Autodesk Inventor part; units mm, degrees
ref_plane "YZ Plane" through (0, 0, 0) normal (1, 0, 0) x (0, 1, 0)
ref_plane "XZ Plane" through (0, 0, 0) normal (0, 1, 0) x (-1, 0, 0)
ref_plane "XY Plane" through (0, 0, 0) normal (0, 0, 1) x (1, 0, 0)
sketch "Boceto1" plane through (0, 0, 0) normal (0, 1, 0) x (-1, 0, 0)
  line L0 (-50, 28) -> (-53, 28)
  line L1 (-50, -28) -> (-50, -22)
  line L2 (-50, -28) -> (-53, -28)
  circle A0 centre (-25, 0) radius 1.5
  circle A1 centre (25, 0) radius 1.5
  line L3 (-53, -25) -> (-53, -28)
  line L4 (-53, -22) -> (-53, -25)
  line L5 (-50, -22) -> (-53, -22)
  line L6 (-50, -28) -> (-50, -22)
  line L7 (-53, -25) -> (-53, -28)
  line L8 (-53, -22) -> (-53, -25)
  line L9 (53, 4.5) -> (53, -4.5)
  line L10 (50, 4.5) -> (53, 4.5)
  line L11 (50, -4.5) -> (50, 4.5)
  line L12 (53, -4.5) -> (50, -4.5)
  line L13 (-50, 22) -> (-50, 28)
  line L14 (-53, 22) -> (-50, 22)
  line L15 (-53, 28) -> (-53, 22)
  line L16 (-50, 28) -> (-53, 28)
  line L17 (19.5, 28) -> (19.5, 25)
  line L18 (6.5, 28) -> (19.5, 28)
  line L19 (6.5, 25) -> (6.5, 28)
  line L20 (19.5, 25) -> (6.5, 25)
  line L21 (56, 31) -> (56, -31)
  line L22 (-56, 31) -> (56, 31)
  line L23 (-56, -31) -> (-56, 31)
  line L24 (56, -31) -> (-56, -31)
  line L25 (-19.5, 28) -> (-19.5, 25)
  line L26 (-6.5, 28) -> (-19.5, 28)
  line L27 (-6.5, 25) -> (-6.5, 28)
  line L28 (-19.5, 25) -> (-6.5, 25)
  line L29 (-19.5, -28) -> (-19.5, -25)
  line L30 (-6.5, -28) -> (-19.5, -28)
  line L31 (-6.5, -25) -> (-6.5, -28)
  line L32 (-19.5, -25) -> (-6.5, -25)
  line L33 (19.5, -25) -> (19.5, -28)
  line L34 (6.5, -25) -> (19.5, -25)
  line L35 (6.5, -28) -> (6.5, -25)
  line L36 (19.5, -28) -> (6.5, -28)
extrude "Extrusión1" add sketch "Boceto1" along normal blind 3
properties part number "Case_Base2" material "MDF Tablero de fibras de densidad media"
Check sheet for the modelled part. Datum: model origin and axes. Units: mm. A direction names the side the tool comes from. Round coordinates to 2 decimals unless told otherwise and drop trailing zeros. Loops run counter-clockwise (first coordinate to the right, second up) from the corner with the lowest first, then second, coordinate; pieces in that order, holes last. Notation, with made-up numbers: M -24,24.25 L -19,24.25 A21 ccw -19,53.25 Z; hole C 4,14 d5. An arc over 180 degrees is marked long. Answer as a JSON object with one key per item and string values.
1. Section check B-B (y = 2.25). State how many separate pieces and enclosed holes the cut face has, plus the area to 3 significant figures.
Reply:
{"separate pieces": "1", "enclosed holes": "9", "area": "6,710 mm²"}
2. Scan lines: line 1 (Z direction, x = 11.5, y = 2.55); line 2 (X direction, y = 0.7, z = -23); line 3 (Z direction, x = 25, y = 1.95). Record each from-to range of solid material in increasing order.
Reply:
{"line 1": "z = -31 to -28, -25 to 25, 28 to 31", "line 2": "x = -56 to 50, 53 to 56", "line 3": "z = -31 to -1.5, 1.5 to 31"}
3. Mould release check, pull along Z, two halves, no side actions. Record for faces 3 (the flat face through (-1, 1, -31)), 4 (the flat face through (-13, 1, 25)), 5 (the flat face through (1, 0, 0)): pulls with the +Z half, pulls with the -Z half, needs draft (parallel to the pull), parting line crosses it, or undercut.
Reply:
{"face 3": "pulls with the -Z half", "face 4": "undercut", "face 5": "needs draft"}
4. Section check A-A (x = -25). Record the boundary of the cut face in (y, z).
Reply:
{"outline": "M 0,-31 L 3,-31 L 3,-1.5 L 0,-1.5 Z; M 0,1.5 L 3,1.5 L 3,31 L 0,31 Z"}
5. Access from +Z, -Z, +X, -X, +Y, -Y to the whole of each face (thin tool, end or side, straight path). Record for faces 1 (the flat face through (-56, 1, 0)), 2 (the flat face through (-13, 1, 28)).
Reply:
{"face 1": "+Z, -Z, -X, +Y, -Y", "face 2": "+Y, -Y"}
